from build123d import *

# Parameters (mm, degrees)
SKETCH_1_R          = 38
EXTRUDE_1_DEPTH     = 8
SKETCH_2_R          = 20
EXTRUDE_2_DEPTH     = 16
SKETCH_7_R          = 22
EXTRUDE_3_DEPTH     = 7
SKETCH_3_R          = 4.5
SKETCH_3_R_2        = 3.25
CUT_EXTRUDE_1_DEPTH = 59.855755878
CUT_EXTRUDE_2_DEPTH = 12
SKETCH_5_R          = 2.25
CUT_EXTRUDE_3_DEPTH = 59.855755878
CUT_EXTRUDE_4_DEPTH = 4


with BuildPart() as part:
    # Эскиз1 → Бобышка-Вытянуть1 (new body)
    with BuildSketch(Plane(origin=(0, 0, 0), x_dir=(1, 0, 0), z_dir=(0, 1, 0))):
        with Locations(Location((0, 0, 0), (0, 0, 270))):
            Circle(SKETCH_1_R)
    extrude(amount=EXTRUDE_1_DEPTH)

    # Эскиз2 → Бобышка-Вытянуть2 (add)
    with BuildSketch(Plane(origin=(0, 8, 0), x_dir=(1, 0, 0), z_dir=(0, 1, 0))):
        with Locations(Location((0, 0, 0), (0, 0, 270))):
            Circle(SKETCH_2_R)
    extrude(amount=EXTRUDE_2_DEPTH)

    # Эскиз7 → Бобышка-Вытянуть3 (add)
    with BuildSketch(Plane(origin=(0, 8, 0), x_dir=(1, 0, 0), z_dir=(0, 1, 0))):
        with Locations(Location((0, 0, 0), (0, 0, 270))):
            Circle(SKETCH_7_R)
    extrude(amount=EXTRUDE_3_DEPTH)

    # Эскиз3 → Вырез-Вытянуть1 (cut, through all)
    with BuildSketch(Plane(origin=(0, 24, 0), x_dir=(1, 0, 0), z_dir=(0, 1, 0))):
        with Locations(Location((0, 14, 0), (0, 0, 270))):
            Circle(SKETCH_3_R)
        with Locations(Location((14, 0, 0), (0, 0, 270))):
            Circle(SKETCH_3_R)
        with Locations(Location((0, -14, 0), (0, 0, 270))):
            Circle(SKETCH_3_R)
        with Locations(Location((-14, 0, 0), (0, 0, 270))):
            Circle(SKETCH_3_R)
        with Locations(Location((0, 0, 0), (0, 0, 270))):
            Circle(SKETCH_3_R_2)
    extrude(amount=-CUT_EXTRUDE_1_DEPTH, mode=Mode.SUBTRACT)

    # Эскиз4 → Вырез-Вытянуть2 (cut)
    with BuildSketch(Plane(origin=(0, 24, 0), x_dir=(1, 0, 0), z_dir=(0, 1, 0))):
        Polygon((5.271310529, -3.109118628), (5.32823098, 3.010529515), (0.056920451, 6.119648143), (-5.271310529, 3.109118628), (-5.32823098, -3.010529515), (-0.056920451, -6.119648143), align=None)
    extrude(amount=-CUT_EXTRUDE_2_DEPTH, mode=Mode.SUBTRACT)

    # Эскиз5 → Вырез-Вытянуть3 (cut, through all)
    with BuildSketch(Plane(origin=(0, 24, 0), x_dir=(1, 0, 0), z_dir=(0, 1, 0))):
        with Locations(Location((0, 32, 0), (0, 0, 270))):
            Circle(SKETCH_5_R)
        with Locations(Location((27.712812921, 16, 0), (0, 0, 270))):
            Circle(SKETCH_5_R)
        with Locations(Location((27.712812921, -16, 0), (0, 0, 270))):
            Circle(SKETCH_5_R)
        with Locations(Location((0, -32, 0), (0, 0, 270))):
            Circle(SKETCH_5_R)
        with Locations(Location((-27.712812921, -16, 0), (0, 0, 270))):
            Circle(SKETCH_5_R)
        with Locations(Location((-27.712812921, 16, 0), (0, 0, 270))):
            Circle(SKETCH_5_R)
    extrude(amount=-CUT_EXTRUDE_3_DEPTH, mode=Mode.SUBTRACT)

    # Эскиз6 → Вырез-Вытянуть4 (cut)
    with BuildSketch(Plane(origin=(0, 8, 0), x_dir=(1, 0, 0), z_dir=(0, 1, 0))):
        Polygon((27.712812921, 11.669872981), (31.462812921, 13.834936491), (31.462812921, 18.165063509), (27.712812921, 20.330127019), (23.962812921, 18.165063509), (23.962812921, 13.834936491), align=None)
        Polygon((3.75, 29.834936491), (3.75, 34.165063509), (0, 36.330127019), (-3.75, 34.165063509), (-3.75, 29.834936491), (0, 27.669872981), align=None)
        Polygon((23.962812921, -18.165063509), (27.712812921, -20.330127019), (31.462812921, -18.165063509), (31.462812921, -13.834936491), (27.712812921, -11.669872981), (23.962812921, -13.834936491), align=None)
        Polygon((-3.75, -29.834936491), (-3.75, -34.165063509), (0, -36.330127019), (3.75, -34.165063509), (3.75, -29.834936491), (0, -27.669872981), align=None)
        Polygon((-27.712812921, -11.669872981), (-31.462812921, -13.834936491), (-31.462812921, -18.165063509), (-27.712812921, -20.330127019), (-23.962812921, -18.165063509), (-23.962812921, -13.834936491), align=None)
        Polygon((-23.962812921, 18.165063509), (-27.712812921, 20.330127019), (-31.462812921, 18.165063509), (-31.462812921, 13.834936491), (-27.712812921, 11.669872981), (-23.962812921, 13.834936491), align=None)
    extrude(amount=-CUT_EXTRUDE_4_DEPTH, mode=Mode.SUBTRACT)


solid = part.part
Can you work these out from the model? Positions are in its coordinate system, mm. A direction names the side the tool comes from. Round coordinates to 2 decimals unless told otherwise and drop trailing zeros. Order: outer loops, then holes, each group sorted by start corner. A loop starts at its lowest first (then second) coordinate and runs counter-clockwise, first axis right, second up. Notation, with made-up numbers: M -13,-33.75 L 9,-33.75 A11 cw 9,-23.75 Z; hole C 59,49.5 d5. An arc over 180 degrees is marked long. Use a Markdown table: item, result.
1) Imagine slicing it at A-A (z = 0). List the corners of the cut face in (x, y) for me.
Geometry says:
| item | result |
|---|---|
| outline | M -38,0 L -18.5,0 L -18.5,24 L -20,24 L -20,15 L -22,15 L -22,8 L -38,8 Z; M -9.5,0 L -3.25,0 L -3.25,12 L -5.3,12 L -5.3,24 L -9.5,24 Z; M 3.25,0 L 9.5,0 L 9.5,24 L 5.3,24 L 5.3,12 L 3.25,12 Z; M 18.5,0 L 38,0 L 38,8 L 22,8 L 22,15 L 20,15 L 20,24 L 18.5,24 Z |
2) Imagine slicing it at D-D (y = 2.25). Give the number of separate pieces and of enclosed holes in the cut face, then the cut area to 3 significant figures.
Geometry says:
| item | result |
|---|---|
| separate pieces | 1 |
| enclosed holes | 11 |
| area | 4,150 mm² |
3) I'm going to push flat-ended pins straight in: P1, Ø2, axis at y = 6, z = 17, coming from the +X side; P2, Ø1, axis at y = 6, z = -9, coming from the +X side; P3, Ø10, axis at x = -11.5, y = 3.5, coming from the -Z side; P4, Ø2, axis at x = -0.5, z = -32.5, coming from the +Y side. Where does each tip first touch, or does it pass through?
Geometry says:
| item | result |
|---|---|
| P1 | stops at x = 34.47 |
| P2 | stops at x = 37.04 |
| P3 | stops at z = -37.44 |
| P4 | passes through |
4) If we mould it in two halves opening along Z, with no side actions, what happens to faces 1 (the face through (0.676, 2.028, -29.854)), 2 (the face through (-8, 0, -1))? For each: +Z half, -Z half, draft (parallel to the pull), parting line (faces both ways), or undercut.
Geometry says:
| item | result |
|---|---|
| face 1 | undercut |
| face 2 | draft |
5) On a 3-axis mill with a long thin cutter (end or side, diameter ignored), from which of +Z, -Z, +X, -X, +Y, -Y can I reach the whole of each face in a straight line? I mean faces 3 (the face through (28.389, 2.028, 18.146)), 4 (the face through (-31.463, 6, 16)). Say none if no direction works.
Geometry says:
| item | result |
|---|---|
| face 3 | +Y, -Y |
| face 4 | +Y |
6) Imagine slicing it at B-B (y = 18). List the corners of the cut face in (x, z) for me.
Geometry says:
| item | result |
|---|---|
| outline | C 0,0 d40; hole C -14,0 d9; hole M -5.33,3.01 L -5.27,-3.11 L 0.06,-6.12 L 5.33,-3.01 L 5.27,3.11 L -0.06,6.12 Z; hole C 0,-14 d9; hole C 0,14 d9; hole C 14,0 d9 |
7) If I drill on line 1 along X through (y, z) = (3.25, 0); line 2 along X through (y, z) = (1.5, 16); line 3 along Y through (x, z) = (-25, -16), over which ranges is the centre line in solid material (lowest first)?
Geometry says:
| item | result |
|---|---|
| line 1 | x = -38 to -18.5, -9.5 to -3.25, 3.25 to 9.5, 18.5 to 38 |
| line 2 | x = -34.47 to -29.96, -25.46 to -4.03, 4.03 to 25.46, 29.96 to 34.47 |
| line 3 | y = 0 to 4 |
8) Imagine slicing it at C-C (x = -16.5). List the corners of the cut face in (y, z) for me.
Geometry says:
| item | result |
|---|---|
| outline | M 0,-34.23 L 8,-34.23 L 8,-14.55 L 15,-14.55 L 15,-11.3 L 24,-11.3 L 24,-3.74 L 0,-3.74 Z; M 0,3.74 L 24,3.74 L 24,11.3 L 15,11.3 L 15,14.55 L 8,14.55 L 8,34.23 L 0,34.23 Z |
